Geometry check sheet. Reference: the model listing, model coordinates, mm. Coordinates: 2 decimals unless noted, no trailing zeros. Write each loop counter-clockwise with the first axis right and the second up, starting at its lowest first coordinate (ties: lowest second). Pieces come first, ordered by that corner, then holes.
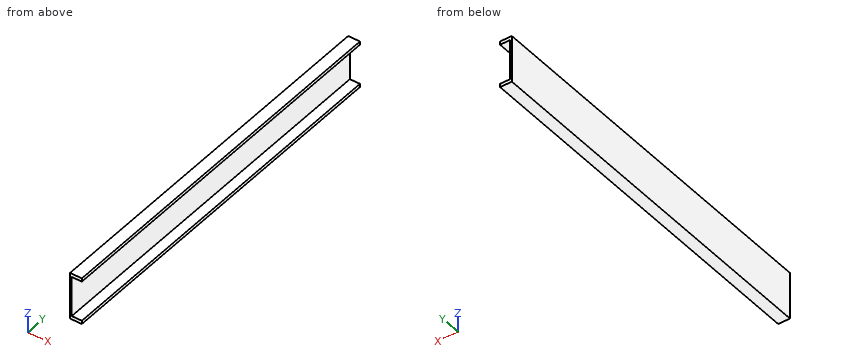
Autodesk Inventor part; units mm, degrees
ref_plane "YZ Plane" through (0, 0, 0) normal (1, 0, 0) x (0, 1, 0)
ref_plane "XZ Plane" through (0, 0, 0) normal (0, 1, 0) x (-1, 0, 0)
ref_plane "XY Plane" through (0, 0, 0) normal (0, 0, 1) x (1, 0, 0)
sketch "Sketch2" plane through (0, 0, 0) normal (0, 1, 0) x (-1, 0, 0)
  line L0 (-5.5563, -22.225) -> (5.5563, -22.225)
  line L1 (5.5563, -22.225) -> (5.5563, 22.225)
  line L2 (5.5563, 22.225) -> (-5.5563, 22.225)
  line L3 (-5.5563, -22.225) -> (5.5563, 22.225) construction
  line L4 (5.5563, -22.225) -> (-5.5563, 22.225) construction
  line L5 (-11.1125, -19.05) -> (1.5875, 19.05) construction
  line L6 (1.5875, -19.05) -> (-11.1125, 19.05) construction
  line L7 (-5.5563, 19.05) -> (-5.5563, 22.225)
  line L8 (-5.5563, -19.05) -> (-5.5563, -22.225)
  line L9 (-5.5563, 19.05) -> (3.9688, 19.05)
  line L10 (3.9688, 19.05) -> (3.9687, -19.05)
  line L11 (3.9687, -19.05) -> (-5.5563, -19.05)
  point P0 (0, 0)
  point P1 (-4.7625, 0)
  dimension "d0" = 11.1125
  dimension "d1" = 44.45
  dimension "d6" = 9.525
  dimension "d7" = 90
extrude "Extrusion1" add sketch "Sketch2" along normal blind 355.6
properties part number "14in-slide-pt_1" material "Aluminum 6061"
1. Thickness scan on line 1 along Z through (x, y) = (-1, 303.5) (3 decimals); line 2 along X through (y, z) = (106.5, -2). Record the ranges inside material, lowest first.
Computed values:
line 1: z = -22.225 to -19.05, 19.05 to 22.225
line 2: x = -5.56 to -3.97
2. Sectioned sample at B-B, the plane y = 273. Record the boundary of the cut face in (x, z) (3 decimals).
Computed values:
outline: (-5.556, -22.225) - (5.556, -22.225) - (5.556, -19.05) - (-3.969, -19.05) - (-3.969, 19.05) - (5.556, 19.05) - (5.556, 22.225) - (-5.556, 22.225) - close
3. Gauge pin test, flat end, axial feed: pin 1 Ø5 at (y, z) = (288.5, 7.5) entering from +X. Record the tip position at first contact, or that the pin passes through.
Computed values:
pin 1: stops at x = -3.97
4. Sectioned sample at C-C, the plane z = 16. Record the boundary of the cut face in (x, y), and give its area (3 significant figures).
Computed values:
outline: (-5.56, 0) - (-3.97, 0) - (-3.97, 355.6) - (-5.56, 355.6) - close
area: 565 mm2
5. Sectioned sample at A-A, the plane x = 2.5. Record the boundary of the cut face in (y, z) (3 decimals).
Computed values:
outline: (0, -22.225) - (355.6, -22.225) - (355.6, -19.05) - (0, -19.05) - close; (0, 19.05) - (355.6, 19.05) - (355.6, 22.225) - (0, 22.225) - close
